The model under review builds one solid part; all positions refer to its coordinate system, in mm. Face numbers are marked on the shaded views. Coordinates: 2 decimals unless noted, no trailing zeros. Write each loop counter-clockwise with the first axis right and the second up, starting at its lowest first coordinate (ties: lowest second). Pieces come first, ordered by that corner, then holes.
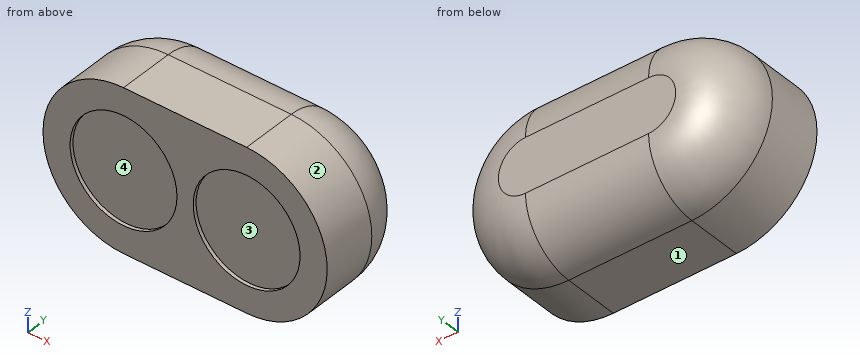
```python
from build123d import *

# Parameters (mm, degrees)
PAD_DEPTH    = 30.48
FILLET_R     = 15
SKETCH001_R  = 15
POCKET_DEPTH = 1


with BuildPart() as part:
    # Sketch → Pad (new body)
    with BuildSketch(Plane.XZ):
        with BuildLine():
            ThreePointArc((-17.272, 22.606), (-39.878, 0), (-17.272, -22.606))
            Line((-17.272, -22.606), (17.272, -22.606))
            ThreePointArc((17.272, -22.606), (39.878, 0), (17.272, 22.606))
            Line((-17.272, 22.606), (17.272, 22.606))
        make_face()
    extrude(amount=PAD_DEPTH)

    # Fillet
    fillet_edges = [part.edges().sort_by_distance(p)[0] for p in [
        (0, 0, 22.606),
    ]]
    fillet(fillet_edges, radius=FILLET_R)

    # Sketch001 (on Face4 of Fillet) → Pocket (cut)
    with BuildSketch(Plane.XZ.offset(30.48)):
        with Locations((-17.272, 0)):
            Circle(SKETCH001_R)
        with Locations((17.272, 0)):
            Circle(SKETCH001_R)
    extrude(amount=-POCKET_DEPTH, mode=Mode.SUBTRACT)


solid = part.part
```
Item 1: For pin 1 (2 mm diameter, centred on x = 30.5, y = -9.5, fed in from -Z); pin 2 (2 mm diameter, centred on y = -24.5, z = -16, fed in from +X); pin 3 (15 mm diameter, centred on x = -24, z = 3, fed in from -Y); pin 4 (24 mm diameter, centred on x = 20.5, z = -4, fed in from -Y), all flat-tipped, find the tip position at first contact; note any pin that passes through.
Solved:
pin 1: stops at z = -17.89
pin 2: stops at x = 34.18
pin 3: stops at y = -29.48
pin 4: stops at y = -30.48
Item 2: Take a section at B-B, the plane y = -23. Write out the cut boundary in (x, z), plus the area to 3 significant figures.
Solved:
outline: (-17.27, -22.61) - (17.27, -22.61) arc R22.61 ccw to (17.27, 22.61) - (-17.27, 22.61) arc R22.61 ccw to start
area: 3,170 mm2
Item 3: Take a section at A-A, the plane x = -13.5. Write out the cut boundary in (y, z).
Solved:
outline: (-30.48, -22.61) - (-15, -22.61) arc R15 ccw to (0, -7.61) - (0, 7.61) arc R15 ccw to (-15, 22.61) - (-30.48, 22.61) - (-30.48, 14.52) - (-29.48, 14.52) - (-29.48, -14.52) - (-30.48, -14.52) - close
Item 4: To check wall thickness, follow line 1 along Y through (x, z) = (-15, -7.5); line 2 along X through (y, z) = (-29, 0); line 3 along X through (y, z) = (-10, 5). State the ranges of each line that lie inside material, in increasing order.
Solved:
line 1: y = -29.48 to 0
line 2: x = -39.88 to 39.88
line 3: x = -38.44 to 38.44
Item 5: Mouldability with a two-part tool opening along X and no side actions: class the marked faces 1, 2, 3 and 4 as pulls with the +X half, pulls with the -X half, needs draft (parallel to the pull), parting line crosses it, or undercut.
Solved:
face 1: needs draft
face 2: pulls with the +X half
face 3: undercut
face 4: undercut
